Verification items for the finished model (mm, model axes). A direction names the side the tool comes from. Round coordinates to 2 decimals unless told otherwise and drop trailing zeros. Write each loop counter-clockwise with the first axis right and the second up, starting at its lowest first coordinate (ties: lowest second). Pieces come first, ordered by that corner, then holes. Notation, with made-up numbers: M 12,13 L 68,13 A16 ccw 68,37 Z; hole C 11,-17.75 d7. An arc over 180 degrees is marked long. Answer in a Markdown table with one row per item. Add a question column.
1. Sectioned sample at C-C on x = -14.5. Record the cut outline in (y, z), plus the area to 3 significant figures.
2. Draft check along Y on faces 1 (the cylindrical face through (2.17, -0.9, 19.68)), 2 (the flat face through (-9, 19, 0)), 3 (the cylindrical face through (-1.507, 6.785, 4.493)). Enter one of: pulls with the +Y half, pulls with the -Y half, needs draft (parallel to the pull), parting line crosses it, or undercut.
3. Sectioned sample at D-D on z = 12.75. Record the cut outline in (x, y), plus the area to 3 significant figures.
4. Sectioned sample at B-B on y = 16. Record the cut outline in (x, z).
5. Set-up check for faces 4 (the flat face through (5, -5, 8)), 5 (the cylindrical face through (23.846, 7.509, 3.944)), 6 (the cylindrical face through (-4.482, 20.183, 1.972)): record each of +Z, -Z, +X, -X, +Y, -Y from which the full face is reachable in a straight line by a thin tool's end or side.
6. Sectioned sample at A-A on z = 3. Record the cut outline in (x, y) (3 decimals).
7. Go/stop test with flat-tipped pins: pin 1 Ø1 at (x, y) = (-18, -5) entering from +Z; pin 2 Ø3 at (x, y) = (8, -13.5) entering from -Z; pin 3 Ø4 at (y, z) = (-6, 25) entering from -X; pin 4 Ø4 at (x, z) = (-14, 6.5) entering from +Y. Record where each tip stops, or that it passes through.
8. Material ranges on probe 1 along Y at (x, z) = (0, 1.9) (3 decimals); probe 2 along Y at (x, z) = (0, 4.35); probe 3 along Z at (x, y) = (9, 12), recorded low to high.
```python
from build123d import *

# Parameters (mm, degrees)
F0_R      = 25
F1_DEPTH  = 8
F2_R      = 20.675
F3_DEPTH  = 4
F4_R      = 6.95
F5_DEPTH  = 1
F6_R      = 6.5
F7_DEPTH  = 3.3
F7_TAPER  = 52
F8_R      = 2.35
F9_DEPTH  = 17
F11_DEPTH = 7.1
F11_TAPER = 1


# Not quite as in the source:
# - a feature names something its author has since deleted; it is built from what else it names


with BuildPart() as f1:
    # F0 (on Top) → F1 (new body)
    with BuildSketch(Plane.XY):
        Circle(F0_R)
    extrude(amount=F1_DEPTH)

    # F2 (on face) → F3 (cut)
    with BuildSketch(Plane(origin=(0, 0, 0), x_dir=(1, 0, 0), z_dir=(0, 0, -1))):
        Circle(F2_R)
    extrude(amount=-F3_DEPTH, mode=Mode.SUBTRACT)

    # F4 (on face) → F5 (cut)
    with BuildSketch(Plane(origin=(0, 0, 4), x_dir=(1, 0, 0), z_dir=(0, 0, -1))):
        Circle(F4_R)
    extrude(amount=-F5_DEPTH, mode=Mode.SUBTRACT)

    # F6 (on face) → F7 (join)
    with BuildSketch(Plane.XY.offset(8)):
        Circle(F6_R)
    extrude(amount=F7_DEPTH, taper=F7_TAPER)

    # F8 (on face) → F9 (join)
    with BuildSketch(Plane.XY.offset(11.3)):
        Circle(F8_R)
    extrude(amount=F9_DEPTH)

    # F10 (on face) → F11 (cut)
    with BuildSketch(Plane.XY.offset(28.3)):
        with BuildLine():
            ThreePointArc((-0.65, 2.2583179581), (0, 2.35), (0.65, 2.2583179581))
            Line((0.65, 2.2583179581), (0.65, 4))
            Line((0.65, 4), (-0.65, 4))
            Line((-0.65, 4), (-0.65, 2.2583179581))
        make_face()
        with BuildLine():
            ThreePointArc((-0.65, -2.2583179581), (0, -2.35), (0.65, -2.2583179581))
            Line((0.65, -2.2583179581), (0.65, 2.2583179581))
            ThreePointArc((0.65, 2.2583179581), (0, 2.35), (-0.65, 2.2583179581))
            Line((-0.65, 2.2583179581), (-0.65, -2.2583179581))
        make_face()
        with BuildLine():
            Line((-0.65, -4), (0.65, -4))
            Line((0.65, -4), (0.65, -2.2583179581))
            ThreePointArc((0.65, -2.2583179581), (0, -2.35), (-0.65, -2.2583179581))
            Line((-0.65, -2.2583179581), (-0.65, -4))
        make_face()
    extrude(amount=-F11_DEPTH, taper=F11_TAPER, mode=Mode.SUBTRACT)


solid = f1.part
```
Geometry check:
| question | item | result |
|---|---|---|
| 1 | outline | M -20.37,0 L -14.74,0 L -14.74,4 L 14.74,4 L 14.74,0 L 20.37,0 L 20.37,8 L -20.37,8 Z |
| 1 | area | 208 mm2 |
| 2 | face 1 | parting line crosses it |
| 2 | face 2 | needs draft |
| 2 | face 3 | undercut |
| 3 | outline | C 0,0 d4.7 |
| 3 | area | 17.3 mm2 |
| 4 | outline | M -19.21,0 L -13.09,0 L -13.09,4 L 13.09,4 L 13.09,0 L 19.21,0 L 19.21,8 L -19.21,8 Z |
| 5 | face 4 | +Z |
| 5 | face 5 | +Z, -Z |
| 5 | face 6 | -Z |
| 6 | outline | C 0,0 d50; hole C 0,0 d41.35 |
| 7 | pin 1 | stops at z = 8 |
| 7 | pin 2 | stops at z = 4 |
| 7 | pin 3 | passes through |
| 7 | pin 4 | stops at y = 21.93 |
| 8 | probe 1 | y = -25 to -20.675, 20.675 to 25 |
| 8 | probe 2 | y = -25 to -6.95, 6.95 to 25 |
| 8 | probe 3 | z = 4 to 8 |
